For this review, take the finished solid that the model builds, in its own axes (mm). A direction names the side the tool comes from. Give positions to 0.01 mm unless a question says otherwise; leave off trailing zeros. Write each loop counter-clockwise with the first axis right and the second up, starting at its lowest first coordinate (ties: lowest second). Pieces come first, ordered by that corner, then holes. Notation, with made-up numbers: (69.25, -19.5) -> (86.25, -19.5) arc R28 ccw to (86.25, 9.5) -> close; hole circle Ø7 at (18.5, -3.5). An arc over 180 degrees is marked (long way). Answer as CSV lines item,"result".
```python
from build123d import *

# Parameters (mm, degrees)
PAD_DEPTH       = 95
SKETCH001_W     = 37
SKETCH001_H     = 15
PAD001_DEPTH    = 2
PAD002_DEPTH    = 2
PAD003_DEPTH    = 2
SKETCH004_W     = 15
SKETCH004_H     = 57
POCKET_DEPTH    = 15.001
SKETCH005_R     = 2.5
POCKET001_DEPTH = 15.001
FILLET_R        = 1
FILLET001_R     = 1
FILLET002_R     = 1
FILLET003_R     = 1
FILLET004_R     = 1
FILLET005_R     = 1
FILLET006_R     = 1
FILLET007_R     = 1
FILLET008_R     = 1
FILLET009_R     = 1


with BuildPart() as part:
    # Sketch → Pad (new body)
    with BuildSketch(Plane.XZ):
        Polygon((2, -3.25), (10, -3.25), (10, 3.25), (0, 3.25), (0, 5.25), (14, 5.25), (14, -7.75), (45, -7.75), (45, 5.25), (47, 5.25), (47, -9.75), (10, -9.75), (10, -5.25), (2, -5.25), align=None)
    extrude(amount=PAD_DEPTH)

    # Sketch001 (on Face15 of Pad) → Pad001 (join)
    with BuildSketch(Plane(origin=(0, 0, 0), x_dir=(1, 0, 0), z_dir=(0, 1, 0))):
        with Locations((28.5, 2.25)):
            Rectangle(SKETCH001_W, SKETCH001_H)
    extrude(amount=-PAD001_DEPTH)

    # Sketch002 (on Face6 of Pad001) → Pad002 (join)
    with BuildSketch(Plane.XZ.offset(95)):
        with BuildLine():
            Line((10, -9.75), (10, -2.75))
            Line((10, -2.75), (18, -2.75))
            ThreePointArc((20, -6.75), (19.553394, -4.473303), (18, -2.75))
            Line((20, -9.75), (20, -6.75))
            Line((10, -9.75), (20, -9.75))
        make_face()
    extrude(amount=-PAD002_DEPTH)

    # Sketch003 (on Face26 of Pad002) → Pad003 (join)
    with BuildSketch(Plane.XZ.offset(95)):
        with BuildLine():
            Line((47, -9.75), (40, -9.75))
            Line((40, -9.75), (40, -5.75))
            ThreePointArc((42, -2.75), (40.644801, -4.013201), (40, -5.75))
            Line((47, -2.75), (42, -2.75))
            Line((47, -9.75), (47, -2.75))
        make_face()
    extrude(amount=-PAD003_DEPTH)

    # Sketch004 (on Face24 of Pad003) → Pocket (cut, through all)
    with BuildSketch(Plane(origin=(0, 0, 5.25), x_dir=(-1, 0, 0), z_dir=(0, 0, 1))):
        with Locations((-7.5, 47.5)):
            Rectangle(SKETCH004_W, SKETCH004_H)
    extrude(amount=-POCKET_DEPTH, mode=Mode.SUBTRACT)

    # Sketch005 (on Face10 of Pocket) → Pocket001 (cut, through all)
    with BuildSketch(Plane(origin=(0, 0, 5.25), x_dir=(-1, 0, 0), z_dir=(0, 0, 1))):
        with Locations((-6, 82)):
            Circle(SKETCH005_R)
        with Locations((-6, 13)):
            Circle(SKETCH005_R)
    extrude(amount=-POCKET001_DEPTH, mode=Mode.SUBTRACT)

    # Fillet
    fillet_edges = [part.edges().sort_by_distance(p)[0] for p in [
        (47, -47.5, -9.75),
    ]]
    fillet(fillet_edges, radius=FILLET_R)

    # Fillet001
    fillet001_edges = [part.edges().sort_by_distance(p)[0] for p in [
        (47, -48.5, 5.25),
    ]]
    fillet(fillet001_edges, radius=FILLET001_R)

    # Fillet002
    fillet002_edges = [part.edges().sort_by_distance(p)[0] for p in [
        (29.5, 0, 5.25),
    ]]
    fillet(fillet002_edges, radius=FILLET002_R)

    # Fillet003
    fillet003_edges = [part.edges().sort_by_distance(p)[0] for p in [
        (10, 0, 0),
    ]]
    fillet(fillet003_edges, radius=FILLET003_R)

    # Fillet004
    fillet004_edges = [part.edges().sort_by_distance(p)[0] for p in [
        (10, 0, -7),
    ]]
    fillet(fillet004_edges, radius=FILLET004_R)

    # Fillet005
    fillet005_edges = [part.edges().sort_by_distance(p)[0] for p in [
        (10, -95, 0.25),
    ]]
    fillet(fillet005_edges, radius=FILLET005_R)

    # Fillet006
    fillet006_edges = [part.edges().sort_by_distance(p)[0] for p in [
        (10, -95, -7.5),
    ]]
    fillet(fillet006_edges, radius=FILLET006_R)

    # Fillet007
    fillet007_edges = [part.edges().sort_by_distance(p)[0] for p in [
        (7, -95, 5.25),
    ]]
    fillet(fillet007_edges, radius=FILLET007_R)

    # Fillet008
    fillet008_edges = [part.edges().sort_by_distance(p)[0] for p in [
        (15, -47.5, -9.75),
    ]]
    fillet(fillet008_edges, radius=FILLET008_R)

    # Fillet009
    fillet009_edges = [part.edges().sort_by_distance(p)[0] for p in [
        (30, -95, -7.75),
    ]]
    fillet(fillet009_edges, radius=FILLET009_R)


solid = part.part
```
Q1. To check wall thickness, follow probe 1 along X at (y, z) = (-82, -3.85); probe 2 along Y at (x, z) = (6, 4.1); probe 3 along Z at (x, y) = (8, -78). State the ranges of each line that lie inside material, in increasing order. Write a range as [from, to].
Answer block:
probe 1,"x = [2, 3.5], [8.5, 14], [45, 47]"
probe 2,"y = [-95, -84.5], [-79.5, -76], [-19, -15.5], [-10.5, 0]"
probe 3,"z = [-5.25, -3.25], [3.25, 5.25]"
Q2. Clearance check with flat-ended pins moving along their axes: pin 1 (3 mm diameter, centred on x = 6, y = -13, fed in from -Z); pin 2 (2 mm diameter, centred on y = -89, z = -8, fed in from -X); pin 3 (2 mm diameter, centred on x = 26, z = -5, fed in from -Y); pin 4 (4.5 mm diameter, centred on x = 4.5, y = -89.5, fed in from -Z). State where each tip first meets the part, or that it passes through.
Answer block:
pin 1,"passes through"
pin 2,"stops at x = 10"
pin 3,"stops at y = -2"
pin 4,"stops at z = -5.25"
Q3. For faces 5 (the flat face through (45, -48, -1)), 6 (the cylindrical face through (3.69, -81.04, 4.26)), 7 (the flat face through (40, -94, -7)), 8 (the flat face through (10, -85, 0)), 9 (the flat face through (10, -10, -7)), list the 3-axis set-ups (+Z, -Z, +X, -X, +Y, -Y) from which the entire face can be reached by the end or side of a thin tool; tool diameter is ignored.
Answer block:
face 5,"+Z"
face 6,"+Z, -Z"
face 7,"+Z, -Y"
face 8,"-X, +Y, -Y"
face 9,"-Z, -X, +Y, -Y"
Q4. Draft analysis for pull direction Z (two halves, no side actions). For faces 1 (the flat face through (6, -85, -5.25)), 2 (the flat face through (4, -9, 3.25)), 3 (the flat face through (7, -85, 5.25)), 4 (the cylindrical face through (4.85, -10.78, -4.24)), state which applies: released by +Z, released by -Z, zero draft, split by the parting line, or undercut.
Answer block:
face 1,"released by -Z"
face 2,"undercut"
face 3,"released by +Z"
face 4,"zero draft"
Q5. Add section D-D (y = -27). Write out the cut boundary in (x, z), plus the area to 3 significant figures.
Answer block:
outline,"(15, -8.75) arc R1 ccw to (16, -9.75) -> (46, -9.75) arc R1 ccw to (47, -8.75) -> (47, 4.25) arc R1 ccw to (46, 5.25) -> (45, 5.25) -> (45, -7.75) -> (15, -7.75) -> close"
area,"89.4 mm2"
Q6. Add section C-C (y = -82). Write out the cut boundary in (x, z).
Answer block:
outline,"(0, 3.25) -> (3.5, 3.25) -> (3.5, 5.25) -> (0, 5.25) -> close; (2, -5.25) -> (3.5, -5.25) -> (3.5, -3.25) -> (2, -3.25) -> close; (8.5, -5.25) -> (10, -5.25) -> (10, -9.75) -> (46, -9.75) arc R1 ccw to (47, -8.75) -> (47, 4.25) arc R1 ccw to (46, 5.25) -> (45, 5.25) -> (45, -7.75) -> (14, -7.75) -> (14, 5.25) -> (8.5, 5.25) -> (8.5, 3.25) -> (10, 3.25) -> (10, -3.25) -> (8.5, -3.25) -> close"
Q7. Add section A-A (x = 6). State how many separate pieces and enclosed holes the cut face has, plus the area to 3 significant figures.
Answer block:
separate pieces,"8"
enclosed holes,"0"
area,"112 mm2"
Q8. Add section B-B (z = -0.75). Write out the cut boundary in (x, y).
Answer block:
outline,"(10, -94) arc R1 ccw to (11, -95) -> (14, -95) -> (14, -76) -> (10, -76) -> close; (10, -19) -> (14, -19) -> (14, -2) -> (45, -2) -> (45, -95) -> (47, -95) -> (47, -1) arc R1 ccw to (46, 0) -> (11, 0) arc R1 ccw to (10, -1) -> close"
